The model under review builds one solid part; all positions refer to its coordinate system, in mm. Round coordinates to 2 decimals unless told otherwise and drop trailing zeros. Order: outer loops, then holes, each group sorted by start corner. A loop starts at its lowest first (then second) coordinate and runs counter-clockwise, first axis right, second up.
```python
from build123d import *

# Parameters (mm, degrees)
SKETCH_1_W          = 95
SKETCH_1_H          = 38.85
EXTRUDE_1_DEPTH     = 0.5
SKETCH_2_W          = 38.85
SKETCH_2_H          = 95
EXTRUDE_2_DEPTH     = 0.5
SKETCH_3_W          = 29.202398915
SKETCH_3_H          = 25.024241253
CUT_EXTRUDE_1_DEPTH = 110.347085009


with BuildPart() as part:
    # Эскиз1 → Бобышка-Вытянуть1 (new body)
    with BuildSketch(Plane(origin=(0.5, 0, 0), x_dir=(0, -1, 0), z_dir=(-1, 0, 0))):
        with Locations((-53.35, 22.825)):
            Rectangle(SKETCH_1_W, SKETCH_1_H)
    extrude(amount=-EXTRUDE_1_DEPTH)

    # Эскиз2 → Бобышка-Вытянуть2 (add)
    with BuildSketch(Plane.ZY.offset(-0.5)):
        with Locations((22.825, 53.35)):
            Rectangle(SKETCH_2_W, SKETCH_2_H)
    extrude(amount=EXTRUDE_2_DEPTH)

    # Эскиз3 → Вырез-Вытянуть1 (cut, through all)
    with BuildSketch(Plane.ZY):
        Polygon((47.187175015, 54.261978396), (29.562288031, 54.261978396), (29.562288031, 50.078726521), (28.618889228, 50.078726521), (28.618889228, 47.878726521), (29.562288031, 47.878726521), (29.562288031, 33.238726521), (28.618889228, 33.238726521), (28.618889228, 31.038726521), (29.562288031, 31.038726521), (29.562288031, 25.969159943), (47.187175015, 25.969159943), align=None)
        with Locations((30.007497179, 83.917054381)):
            Rectangle(SKETCH_3_W, SKETCH_3_H)
    extrude(amount=-CUT_EXTRUDE_1_DEPTH, mode=Mode.SUBTRACT)


solid = part.part
```
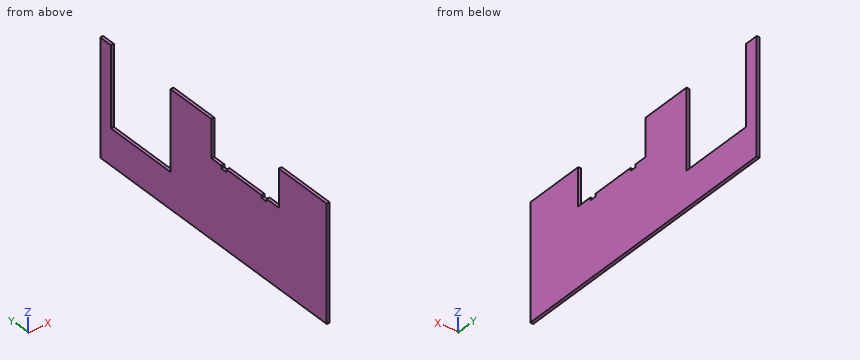
(1) Insertion check: pin 1 (0.5 mm diameter, centred on x = 0.5, y = 52.5, fed in from +Z). The pin has a flat end and moves straight along its axis. Give the tip position at first contact, or say it passes through.
Data:
pin 1: stops at z = 29.56
(2) To check wall thickness, follow probe 1 along Y at (x, z) = (0.95, 34); probe 2 along Y at (x, z) = (0.25, 28); probe 3 along Z at (x, y) = (0.3, 50). State the ranges of each line that lie inside material, in increasing order.
Data:
probe 1: y = 5.85 to 25.97, 54.26 to 71.4, 96.43 to 100.85
probe 2: y = 5.85 to 71.4, 96.43 to 100.85
probe 3: z = 3.4 to 28.62
(3) Consider section D-D (y = 46). Write out the cut boundary in (x, z), and give its area (3 significant figures).
Data:
outline: (0, 3.4) - (1, 3.4) - (1, 29.56) - (0, 29.56) - close
area: 26.2 mm2
(4) Consider section B-B (x = 0.5). Write out the cut boundary in (y, z).
Data:
outline: (5.85, 3.4) - (100.85, 3.4) - (100.85, 42.25) - (96.43, 42.25) - (96.43, 15.41) - (71.4, 15.41) - (71.4, 42.25) - (54.26, 42.25) - (54.26, 29.56) - (50.08, 29.56) - (50.08, 28.62) - (47.88, 28.62) - (47.88, 29.56) - (33.24, 29.56) - (33.24, 28.62) - (31.04, 28.62) - (31.04, 29.56) - (25.97, 29.56) - (25.97, 42.25) - (5.85, 42.25) - close
(5) Consider section A-A (z = 32). Write out the cut boundary in (x, y).
Data:
outline: (0, 5.85) - (1, 5.85) - (1, 25.97) - (0, 25.97) - close; (0, 54.26) - (1, 54.26) - (1, 71.4) - (0, 71.4) - close; (0, 96.43) - (1, 96.43) - (1, 100.85) - (0, 100.85) - close
(6) Consider section C-C (z = 26). Write out the cut boundary in (x, y).
Data:
outline: (0, 5.85) - (1, 5.85) - (1, 71.4) - (0, 71.4) - close; (0, 96.43) - (1, 96.43) - (1, 100.85) - (0, 100.85) - close
